Source: CAD feature listing. Evaluate the final solid. Frame: model axes, mm. A direction names the side the tool comes from. Round coordinates to 2 decimals unless told otherwise and drop trailing zeros. Write each loop counter-clockwise with the first axis right and the second up, starting at its lowest first coordinate (ties: lowest second). Pieces come first, ordered by that corner, then holes.
from build123d import *

# Parameters (mm, degrees)
F0_R     = 75.838692
F1_DEPTH = 177.8
F2_R     = 61.132843
F4_DEPTH = 215.9
F3_R     = 17.420923
F5_DEPTH = 215.9
F6_R     = 67.546104
F7_DEPTH = 101.6
F8_R     = 58.022008
F9_DEPTH = 406.4


with BuildPart() as f1:
    # F0 (on Front) → F1 (new body)
    with BuildSketch(Plane.XZ):
        Circle(F0_R)
    extrude(amount=F1_DEPTH)

    # F2 (on Front) → F4 (join)
    with BuildSketch(Plane.XZ):
        Circle(F2_R)
    extrude(amount=F4_DEPTH)

    # F3 (on Front) → F5 (cut)
    with BuildSketch(Plane.XZ):
        Circle(F3_R)
    extrude(amount=F5_DEPTH, mode=Mode.SUBTRACT)

    # F6 (on Front) → F7 (cut)
    with BuildSketch(Plane.XZ):
        Circle(F6_R)
    extrude(amount=F7_DEPTH, mode=Mode.SUBTRACT)

    # F8 (on Front) → F9 (join)
    with BuildSketch(Plane.XZ):
        Circle(F8_R)
    extrude(amount=F9_DEPTH)


solid = f1.part
1) Section query D-D on y = -291. Return the cut outline in (x, z).
Taken from the geometry:
outline: circle Ø116.04 at (0, 0)
2) Reachability of faces 1 (the face through (-51, -177.8, 34)), 2 (the face through (31.168, -50.089, -59.925)), 3 (the face through (-1, -406.4, 1)) from +Z, -Z, +X, -X, +Y, -Y: full face, straight path, thin tool, end or side. Return the list, or none.
Taken from the geometry:
face 1: -Y
face 2: +Y
face 3: +Z, -Z, +X, -X, -Y
3) Pull-direction query (X, two-part tool) for faces 4 (the face through (-12.58, -309.82, -56.64)), 5 (the face through (-51, 0, -45)), 6 (the face through (30, -101.6, 50)), 7 (the face through (-12.58, -50.09, -56.64)); classes: released by +X, released by -X, zero draft, split by the parting line, or undercut.
Taken from the geometry:
face 4: split by the parting line
face 5: zero draft
face 6: undercut
face 7: undercut
4) Section query C-C on y = -128. Return the cut outline in (x, z).
Taken from the geometry:
outline: circle Ø151.68 at (0, 0)
5) Section query A-A on x = 0. Return the cut outline in (y, z).
Taken from the geometry:
outline: (-406.4, -58.02) - (-215.9, -58.02) - (-215.9, -61.13) - (-177.8, -61.13) - (-177.8, -75.84) - (0, -75.84) - (0, -67.55) - (-101.6, -67.55) - (-101.6, -58.02) - (0, -58.02) - (0, 58.02) - (-101.6, 58.02) - (-101.6, 67.55) - (0, 67.55) - (0, 75.84) - (-177.8, 75.84) - (-177.8, 61.13) - (-215.9, 61.13) - (-215.9, 58.02) - (-406.4, 58.02) - close
6) Material intervals for line 1 (Z direction, x = 0, y = -69.5); line 2 (X direction, y = -94, z = -28); line 3 (X direction, y = -24, z = 4.5), sorted ascending.
Taken from the geometry:
line 1: z = -75.84 to -67.55, -58.02 to 58.02, 67.55 to 75.84
line 2: x = -70.48 to -61.47, -50.82 to 50.82, 61.47 to 70.48
line 3: x = -75.71 to -67.4, -57.85 to 57.85, 67.4 to 75.71
7) Contact query for flat-ended pins moving along their axis: P1, Ø2, axis at x = -42, y = -320.5, coming from the +Z side; P2, Ø12, axis at x = -2, y = -290.5, coming from the -Z side; P3, Ø5, axis at x = 23.5, y = -114.5, coming from the +Z side. Output: stop coordinate, or through.
Taken from the geometry:
P1: stops at z = 41.06
P2: stops at z = -58.02
P3: stops at z = 72.87
8) Section query B-B on z = 0. Return the cut outline in (x, y), then the cut area to 3 significant figures.
Taken from the geometry:
outline: (-75.84, -177.8) - (-61.13, -177.8) - (-61.13, -215.9) - (-58.02, -215.9) - (-58.02, -406.4) - (58.02, -406.4) - (58.02, -215.9) - (61.13, -215.9) - (61.13, -177.8) - (75.84, -177.8) - (75.84, 0) - (67.55, 0) - (67.55, -101.6) - (58.02, -101.6) - (58.02, 0) - (-58.02, 0) - (-58.02, -101.6) - (-67.55, -101.6) - (-67.55, 0) - (-75.84, 0) - close
area: 51,800 mm2
